Geometry check sheet. Reference: the model listing, model coordinates, mm. Face numbers are marked on the shaded views. A direction names the side the tool comes from. Round coordinates to 2 decimals unless told otherwise and drop trailing zeros. Loops run counter-clockwise (first coordinate to the right, second up) from the corner with the lowest first, then second, coordinate; pieces in that order, holes last.
```python
from build123d import *
from build123d.topology import SkipClean

# Parameters (mm, degrees)
BOSS_EXTRUDE1_DEPTH = 2
SKETCH2_W           = 31
SKETCH2_H           = 28
BOSS_EXTRUDE2_DEPTH = 2
BOSS_EXTRUDE3_DEPTH = 4
CUT_EXTRUDE1_DEPTH  = 4
FILLET1_R           = 1
CUT_EXTRUDE2_START  = -29
SKETCH5_R           = 4
CUT_EXTRUDE2_DEPTH  = 10
SKETCH6_R           = 2.5
CUT_EXTRUDE3_DEPTH  = 10
SCALE1_SCALE        = 0.5


with BuildPart() as part:
    # Sketch1 → Boss-Extrude1 (new body)
    with BuildSketch(Plane(origin=(0, 0, 0), x_dir=(0, 0, -1), z_dir=(1, 0, 0))):
        with BuildLine():
            Line((-6.709990017, 1.993999493), (3.096579457, 34.993999493))
            Line((3.096579457, 34.993999493), (3.096579457, 36.993999493))
            Line((3.096579457, 36.993999493), (31.096579457, 36.993999493))
            Line((31.096579457, 36.993999493), (31.096579457, 31.032332545))
            ThreePointArc((31.096579457, 31.032332545), (30.777696783, 29.102331009), (29.854944147, 27.377477489))
            Line((29.854944147, 27.377477489), (5.551425471, -4.263997566))
            ThreePointArc((5.551425471, -4.263997566), (-3.182169032, -6.234885745), (-6.709990017, 1.993999493))
        make_face()
    extrude(amount=-BOSS_EXTRUDE1_DEPTH)


with BuildPart() as body_2:
    # Mirror1: mirrored copy
    add(part.part.mirror(Plane(origin=(-15.5, 0, 0), x_dir=(0, 0, 1), z_dir=(1, 0, 0))))


with BuildPart() as part_1:
    add(part.part)

    add(body_2.part)  # Boss-Extrude2 merges body 2
    # Sketch2 → Boss-Extrude2 (add)
    with BuildSketch(Plane(origin=(0, 36.993999493, 0), x_dir=(1, 0, 0), z_dir=(0, 1, 0))):
        with Locations((-15.5, 17.096579457)):
            Rectangle(SKETCH2_W, SKETCH2_H)
    extrude(amount=-BOSS_EXTRUDE2_DEPTH)

    # Sketch3 → Boss-Extrude3 (add)
    with BuildSketch(Plane(origin=(0, 36.993999493, 0), x_dir=(1, 0, 0), z_dir=(0, 1, 0))):
        with BuildLine():
            Line((-7.41958555, 31.09226783), (-5.143842411, 31.096579457))
            ThreePointArc((-5.143842411, 31.096579457), (-15.5, 14.596579457), (-25.856157589, 31.096579457))
            Line((-25.856157589, 31.096579457), (-23.58041445, 31.09226783))
            ThreePointArc((-23.58041445, 31.09226783), (-15.5, 16.596579457), (-7.41958555, 31.09226783))
        make_face()
    extrude(amount=-BOSS_EXTRUDE3_DEPTH)

    # Sketch4 → Cut-Extrude1 (cut)
    with SkipClean():  # the faces are left unmerged after this step: merging them gives an invalid solid
        with BuildSketch(Plane.XZ.offset(-34.993999493)):
            with BuildLine():
                Line((-5.143842411, -31.096579457), (-7.41958555, -31.09226783))
                ThreePointArc((-7.41958555, -31.09226783), (-15.5, -16.596579457), (-23.58041445, -31.09226783))
                Line((-23.58041445, -31.09226783), (-25.856157589, -31.096579457))
                Line((-25.856157589, -31.096579457), (-5.143842411, -31.096579457))
            make_face()
        extrude(amount=-CUT_EXTRUDE1_DEPTH, mode=Mode.SUBTRACT)

    # Fillet1
    fillet1_edges = [part_1.edges().sort_by_distance(p)[0] for p in [
        (-31, 36.993999493, -17.096579457),
        (0, 36.993999493, -17.096579457),
    ]]
    fillet(fillet1_edges, radius=FILLET1_R)

    # Sketch5 → Cut-Extrude2 (cut)
    with SkipClean():  # the faces are left unmerged after this step: merging them gives an invalid solid
        with BuildSketch(Plane(origin=(0, 0, 0), x_dir=(0, 0, -1), z_dir=(1, 0, 0)).offset(CUT_EXTRUDE2_START)):
            with Locations(Location((0, 0, 0), (0, 0, 180))):
                Circle(SKETCH5_R)
        extrude(amount=-CUT_EXTRUDE2_DEPTH, mode=Mode.SUBTRACT)

    # Sketch6 → Cut-Extrude3 (cut)
    with SkipClean():  # the faces are left unmerged after this step: merging them gives an invalid solid
        with BuildSketch(Plane(origin=(0, 0, 0), x_dir=(0, 0, -1), z_dir=(1, 0, 0))):
            Circle(SKETCH6_R)
        extrude(amount=-CUT_EXTRUDE3_DEPTH, mode=Mode.SUBTRACT)


with BuildPart() as part_2:
    # Scale1: scaled about (0, 0, 0)
    add(part_1.part.scale(SCALE1_SCALE))


solid = part_2.part
```
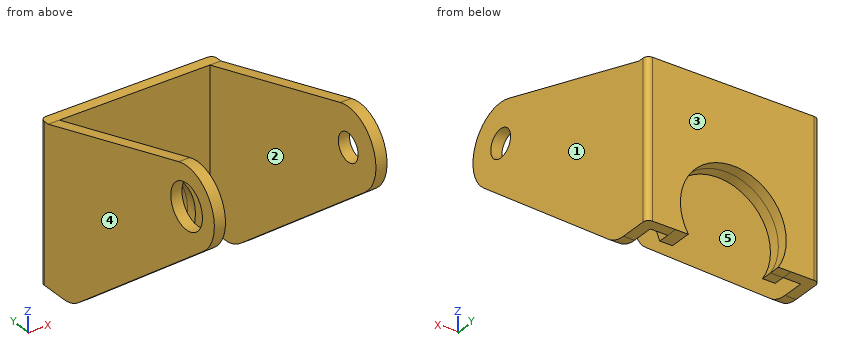
1) Gauge pin test, flat ends, axial feed: pin 1 (1.5 mm diameter, centred on y = 0, z = 0, fed in from +X); pin 2 (4 mm diameter, centred on x = -14, y = 10.5, fed in from -Z); pin 3 (0.5 mm diameter, centred on x = -5.5, y = 18, fed in from +Z). Record the tip position at first contact, or that the pin passes through.
Report:
pin 1: passes through
pin 2: stops at z = -13.97
pin 3: stops at z = -1.55
2) Sectioned sample at A-A, the plane z = -0.25. Record the cut outline in (x, y).
Report:
outline: (-15.5, -3.49) - (-14.5, -3.49) - (-14.5, -1.98) - (-15.5, -1.98) - close; (-15.5, 1.98) - (-14.5, 1.98) - (-14.5, 13.13) - (-15.5, 13.13) - close; (-1, -3.49) - (0, -3.49) - (0, -1.22) - (-1, -1.22) - close; (-1, 1.22) - (0, 1.22) - (0, 13.13) - (-1, 13.13) - close
3) Sectioned sample at C-C, the plane x = -7.75. Record the cut outline in (y, z), then the cut area to 3 significant figures.
Report:
outline: (16.5, -8.3) - (18.5, -8.3) - (18.5, -1.55) - (17.5, -1.55) - (17.5, -7.3) - (16.5, -7.3) - close
area: 7.75 mm2
4) Sectioned sample at B-B, the plane y = 4.5. Record the cut outline in (x, z), then the cut area to 3 significant figures.
Report:
outline: (-15.5, -7.87) - (-14.5, -7.87) - (-14.5, 2.31) - (-15.5, 2.31) - close; (-1, -7.87) - (0, -7.87) - (0, 2.31) - (-1, 2.31) - close
area: 20.4 mm2
5) Access from +Z, -Z, +X, -X, +Y, -Y to the whole of each face (thin tool, end or side, straight path). Record for the marked faces 1 and 2.
Report:
face 1: +Z, -Z, +X, +Y, -Y
face 2: +Z, -Z, -Y
6) Sectioned sample at D-D, the plane y = 0. Record the cut outline in (x, z).
Report:
outline: (-15.5, -4.41) - (-14.5, -4.41) - (-14.5, -2) - (-15.5, -2) - close; (-15.5, 2) - (-14.5, 2) - (-14.5, 3.5) - (-15.5, 3.5) - close; (-1, -4.41) - (0, -4.41) - (0, -1.25) - (-1, -1.25) - close; (-1, 1.25) - (0, 1.25) - (0, 3.5) - (-1, 3.5) - close
7) Mould release check, pull along X, two halves, no side actions. Record for the marked faces 3, 4 and 5: +X half, -X half, draft (parallel to the pull), parting line (faces both ways), or undercut.
Report:
face 3: draft
face 4: -X half
face 5: undercut
8) Scan lines: line 1 along X through (y, z) = (7.5, -5.75); line 2 along Y through (x, z) = (-1.5, -10.75); line 3 along Z through (x, y) = (-7.75, 16.75). Record each from-to range of solid material in increasing order.
Report:
line 1: x = -15.5 to -14.5, -1 to 0
line 2: y = 17.5 to 18.5
line 3: z = -8.3 to -7.3
